The figure shows three views and two pictorial views of one solid part (mm, origin at its lowest corner). Answer the questions. A direction names the side the tool comes from. Coordinates: 2 decimals unless noted, no trailing zeros. Order: outer loops, then holes, each group sorted by start corner. A loop starts at its lowest first (then second) coordinate and runs counter-clockwise, first axis right, second up. Notation, with made-up numbers: (-21.5, 36) - (35.5, 36) arc R15 cw to (35.5, 40) - close; hole circle Ø3 at (-3, 33.5). An arc over 180 degrees is marked (long way). Use one line per item in the form item = value.
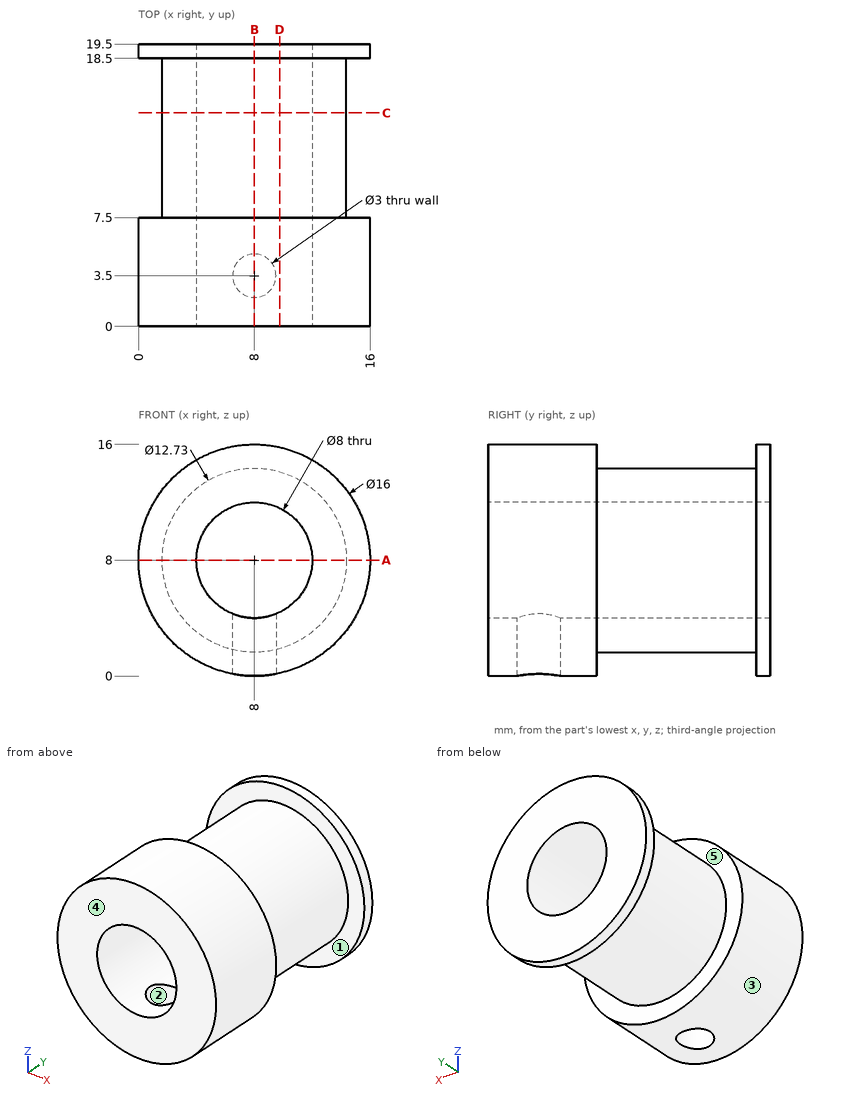
(1) Given pin 1 Ø2 at (x, y) = (14, 3) entering from -Z (3 decimals); pin 2 Ø2.5 at (x, y) = (8, 3.5) entering from -Z; pin 3 Ø1.5 at (x, y) = (5, 13.5) entering from +Z; pin 4 Ø5 at (x, z) = (8, 8) entering from -Y, each flat-ended and moving along its own axis, determine where each tip first touches the part or whether it passes through.
Answer list:
pin_1 = 1.755
pin_2 = 11.8
pin_3 = 13.95
pin_4 = through
(2) Section B-B, the plane x = 8 is taken. Write down the section's boundary in (y, z) (3 decimals), then the cut area to 3 significant figures.
Answer list:
outline = (0, 0) - (2, 0) - (2, 4) - (0, 4) - close; (0, 12) - (19.5, 12) - (19.5, 16) - (18.5, 16) - (18.5, 14.365) - (7.5, 14.365) - (7.5, 16) - (0, 16) - close; (5, 0) - (7.5, 0) - (7.5, 1.635) - (18.5, 1.635) - (18.5, 0) - (19.5, 0) - (19.5, 4) - (5, 4) - close
area = 108 mm2
(3) Which of the six approach directions +Z, -Z, +X, -X, +Y, -Y give full straight-line access (tool end or side, diameter ignored) to the marked faces 4 and 5?
Answer list:
face_4 = +Z, -Z, +X, -X, -Y
face_5 = none
(4) Straight lines are drawn through the part: L1, parallel to Y at x = 8, z = 1.6; L2, parallel to Z at x = 8, y = 9 (3 decimals); L3, parallel to Y at x = 8, z = 2.4. For each, find the intervals that lie inside material, in ascending order.
Answer list:
L1 = 0 to 2, 5 to 7.5, 18.5 to 19.5
L2 = 1.635 to 4, 12 to 14.365
L3 = 0 to 2, 5 to 19.5
(5) Section D-D, the plane x = 9.75 is taken. Write down the section's boundary in (y, z).
Answer list:
outline = (0, 0.19) - (7.5, 0.19) - (7.5, 1.88) - (18.5, 1.88) - (18.5, 0.19) - (19.5, 0.19) - (19.5, 4.4) - (0, 4.4) - close; (0, 11.6) - (19.5, 11.6) - (19.5, 15.81) - (18.5, 15.81) - (18.5, 14.12) - (7.5, 14.12) - (7.5, 15.81) - (0, 15.81) - close
(6) Section A-A, the plane z = 8 is taken. Write down the section's boundary in (x, y) (3 decimals), then the cut area to 3 significant figures.
Answer list:
outline = (0, 0) - (4, 0) - (4, 19.5) - (0, 19.5) - (0, 18.5) - (1.635, 18.5) - (1.635, 7.5) - (0, 7.5) - close; (12, 0) - (16, 0) - (16, 7.5) - (14.365, 7.5) - (14.365, 18.5) - (16, 18.5) - (16, 19.5) - (12, 19.5) - close
area = 120 mm2
(7) The mould has two halves that part along X. Classify the marked faces 1, 2 and 3: +X half, -X half, draft (parallel to the pull), parting line (faces both ways), or undercut.
Answer list:
face_1 = draft
face_2 = undercut
face_3 = parting line
(8) Section C-C, the plane y = 14.75 is taken. Write down the section's boundary in (x, z) (3 decimals), then the cut area to 3 significant figures.
Answer list:
outline = circle Ø12.73 at (8, 8); hole circle Ø8 at (8, 8)
area = 77.0 mm2
